Source: CAD feature listing. Evaluate the final solid. Frame: model axes, mm. Round coordinates to 2 decimals unless told otherwise and drop trailing zeros. Write each loop counter-clockwise with the first axis right and the second up, starting at its lowest first coordinate (ties: lowest second). Pieces come first, ordered by that corner, then holes. Notation, with made-up numbers: M 29.5,53 L 34.5,53 A11 cw 34.5,62 Z; hole C 54.5,80.5 d3. An arc over 180 degrees is marked long. Put each result on its own line as item: value. Start each with the question number.
```python
from build123d import *

# Parameters (mm, degrees)
MAIN_SHAPE_DEPTH                = 6.35
F_1_4_0_25_DIAMETER_HOLE1_D     = 6.35
F_1_4_0_25_DIAMETER_HOLE1_DEPTH = 18
F_1_4_0_25_DIAMETER_HOLE1_TIP   = 1.907732465


with BuildPart() as part:
    # Sketch1 → main shape (new body)
    with BuildSketch(Plane.XY):
        with BuildLine():
            Line((0, 0), (30, 0))
            Line((30, 0), (30, 30))
            ThreePointArc((30, 30), (15, 45), (0, 30))
            Line((0, 30), (0, 0))
        make_face()
    extrude(amount=MAIN_SHAPE_DEPTH)

    # 1/4 (0.25) Diameter Hole1
    with Locations(Plane.XY.offset(6.35)):
        with Locations((15, 30)):
            Hole(F_1_4_0_25_DIAMETER_HOLE1_D / 2, depth=F_1_4_0_25_DIAMETER_HOLE1_DEPTH)
            with Locations((0, 0, -(F_1_4_0_25_DIAMETER_HOLE1_DEPTH + F_1_4_0_25_DIAMETER_HOLE1_TIP / 2))):  # 118° drill point
                Cone(0, F_1_4_0_25_DIAMETER_HOLE1_D / 2, F_1_4_0_25_DIAMETER_HOLE1_TIP, mode=Mode.SUBTRACT)


solid = part.part
```
(1) Section query C-C (y = 41.5). Return loops of the section in (x, z).
(2) Section query B-B (z = 3). Return loops of the section in (x, y) (3 decimals), and give its area (3 significant figures).
(3) Section query A-A (x = 15). Return loops of the section in (y, z) (3 decimals).
(4) Pull-direction query (X, two-part tool) for faces 1 (the flat face through (15, 0, 3)), 2 (the cylindrical face through (13.5, 27.2, 3.1)), 3 (the cylindrical face through (15, 45, 3)); classes: +X half, -X half, draft (parallel to the pull), parting line (faces both ways), or undercut.
(5) Ray query, line 1 along Y through (x, z) = (15, 3) (3 decimals); line 2 along X through (y, z) = (29, 5.25); line 3 along X through (y, z) = (27.5, 3.5). Return the intervals inside material, ascending.
(6) Contact query for flat-ended pins moving along their axis: P1, Ø1, axis at x = 5.5, y = 19, coming from the -Z side; P2, Ø1.5, axis at x = 9.5, z = 4, coming from the +Y side. Output: stop coordinate, or through.
(7) Section query D-D (x = 9.25). Return loops of the section in (y, z), and give its area (3 significant figures).
Entries:
1. outline: M 5.37,0 L 24.63,0 L 24.63,6.35 L 5.37,6.35 Z
2. outline: M 0,0 L 30,0 L 30,30 A15 ccw 0,30 Z; hole C 15,30 d6.35
2. area: 1,220 mm2
3. outline: M 0,0 L 26.825,0 L 26.825,6.35 L 0,6.35 Z; M 33.175,0 L 45,0 L 45,6.35 L 33.175,6.35 Z
4. face 1: draft
4. face 2: undercut
4. face 3: parting line
5. line 1: 0 to 26.825, 33.175 to 45
5. line 2: 0 to 11.99, 18.01 to 30
5. line 3: 0 to 13.04, 16.96 to 30
6. P1: z = 0
6. P2: y = 44.23
7. outline: M 0,0 L 43.85,0 L 43.85,6.35 L 0,6.35 Z
7. area: 278 mm2
